The figure shows three views and two pictorial views of one solid part (mm, origin at its lowest corner). Answer the questions. A direction names the side the tool comes from. Coordinates: 2 decimals unless noted, no trailing zeros. Write each question's results on one line, items separated by ' | '. Start each with the question number.
Item 1: This flat-tipped pin is pushed along its axis until it touches: pin 1 Ø6 at (x, y) = (7.5, 12) entering from -Z. Where does it stop, or does it pass through?
Item 2: Consider probe 1 along Y at (x, z) = (8.75, 4); probe 2 along X at (y, z) = (7.5, 9.75); probe 3 along Y at (x, z) = (11, 4). Determine where each line is inside the solid, lowest interval first. Write a range as [from, to].
Item 3: A tool of negligible diameter and unlimited length cuts with its end or side. For the marked faces 4 and 5, from which of +Z, -Z, +X, -X, +Y, -Y can it reach the whole face along a straight path? Write none if from no direction.
Item 4: For a pull along Y with two mould halves and no side action, classify the marked faces 1, 2 and 3 as +Y half, -Y half, draft (parallel to the pull), parting line (faces both ways), or undercut.
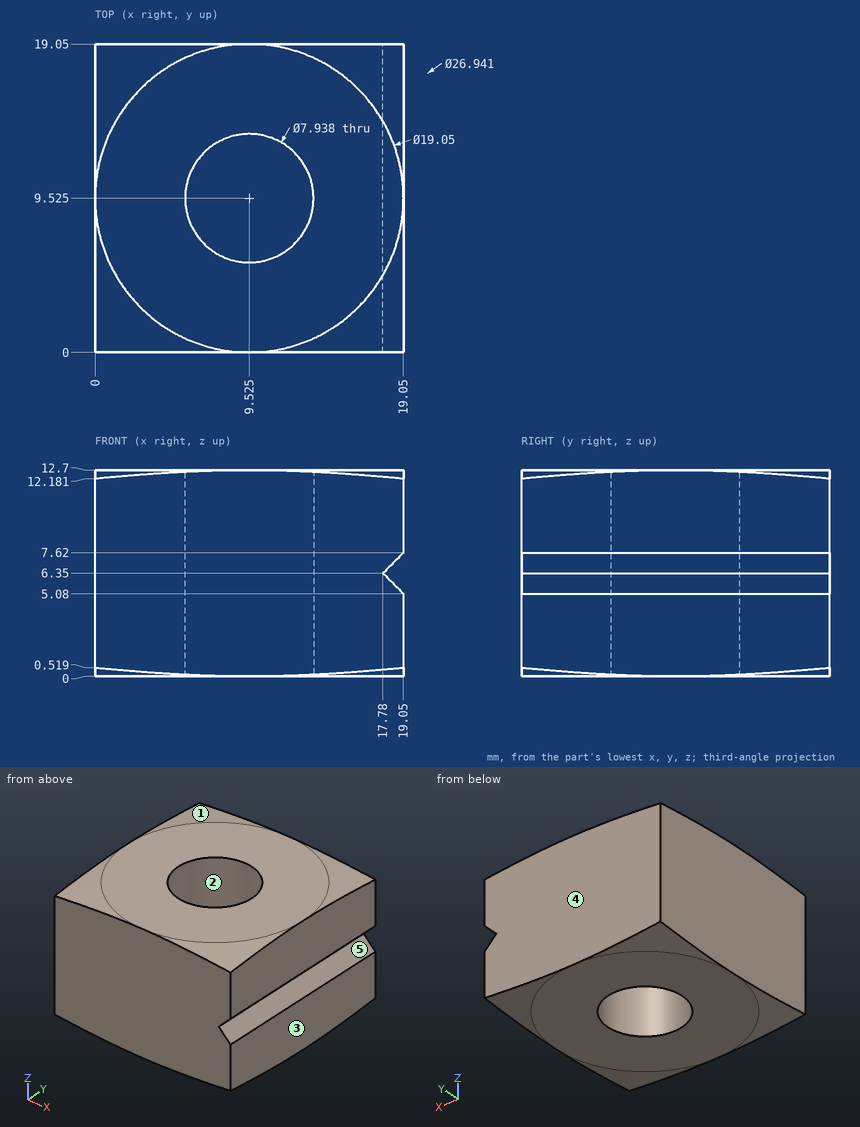
Answer key:
1) pin 1: stops at z = 0
2) probe 1: y = [0, 5.63], [13.42, 19.05] | probe 2: x = [0, 6.11], [12.94, 19.05] | probe 3: y = [0, 5.84], [13.21, 19.05]
3) face 4: +Z, -Z, +X, -X, +Y | face 5: +X, +Y, -Y
4) face 1: +Y half | face 2: undercut | face 3: draft
